from build123d import *

# Parameters (mm, degrees)
BOSS_EXTRUDE2_DEPTH      = 76.2
BOSS_EXTRUDE2_DEPTH_BACK = 76.2
SKETCH3_R                = 6.35
CUT_EXTRUDE5_DEPTH       = 77.727341932
CUT_EXTRUDE5_DEPTH_BACK  = 77.727341932
CHAMFER1_SIZE            = 0.635


with BuildPart() as part:
    # Sketch3 → Boss-Extrude2 (new, two sides: drawn at the far end of the back side and taken through both)
    with BuildSketch(Plane.XY.offset(-BOSS_EXTRUDE2_DEPTH_BACK)):
        with Locations(Location((0, 0, 0), (0, 0, 180))):
            Circle(SKETCH3_R)
    extrude(amount=BOSS_EXTRUDE2_DEPTH + BOSS_EXTRUDE2_DEPTH_BACK)

    # Sketch10 → Cut-Extrude5 (cut, two sides: drawn at the far end of the back side and taken through both)
    with BuildSketch(Plane.XY.offset(-CUT_EXTRUDE5_DEPTH_BACK)):
        with BuildLine():
            Line((-3.175, 5.499261314), (3.175, 5.499261314))
            ThreePointArc((3.175, 5.499261314), (0, 6.35), (-3.175, 5.499261314))
        make_face()
    extrude(amount=CUT_EXTRUDE5_DEPTH + CUT_EXTRUDE5_DEPTH_BACK, mode=Mode.SUBTRACT)

    # Chamfer1
    chamfer1_edges = [part.edges().sort_by_distance(p)[0] for p in [
        (0, -6.35, -76.2),
        (0, -6.35, 76.2),
    ]]
    chamfer(chamfer1_edges, length=CHAMFER1_SIZE)


solid = part.part
Input: part model. Units: mm. Frame: model coordinates. Coordinates: 2 decimals unless noted, no trailing zeros. Loops run counter-clockwise (first coordinate to the right, second up) from the corner with the lowest first, then second, coordinate; pieces in that order, holes last.
Q1. Material intervals for line 1 (Y direction, x = -2.75, z = 30); line 2 (X direction, y = -2.75, z = -5.5); line 3 (Y direction, x = -0.25, z = -67), sorted ascending.
Q2. Cut plane A-A (z = -66). Output: boundary loops of the cut face in (x, y) (3 decimals).
Q3. Contact query for flat-ended pins moving along their axis: pin 1 (1 mm diameter, centred on y = 2, z = -43, fed in from +X); pin 2 (2 mm diameter, centred on y = 3, z = 8, fed in from -X); pin 3 (1.5 mm diameter, centred on x = 5, z = 6, fed in from -Y). Output: stop coordinate, or through.
Working result:
1. line 1: y = -5.72 to 5.5
1. line 2: x = -5.72 to 5.72
1. line 3: y = -6.35 to 5.5
2. outline: (-3.175, 5.499) arc R6.35 ccw (long way) to (3.175, 5.499) - close
3. pin 1: stops at x = 6.17
3. pin 2: stops at x = -6.03
3. pin 3: stops at y = -4.72
